from build123d import *

# Parameters (mm, degrees)
F1_DEPTH = 60


with BuildPart() as f1:
    # F0 (on Top) → F1 (new body)
    with BuildSketch(Plane.XY):
        with BuildLine():
            Line((-85, -85), (85, -85))
            Line((85, -85), (83.56066, -83.56066))
            ThreePointArc((83.56066, -83.56066), (81.43934, -83.56066), (81.43934, -81.43934))
            Line((81.43934, -81.43934), (80.000001, -80.000001))
            Line((80.000001, -80.000001), (-80.000001, -80.000001))
            Line((-80.000001, -80.000001), (-81.43934, -81.43934))
            ThreePointArc((-81.43934, -81.43934), (-81.114181, -81.925975), (-81, -82.5))
            ThreePointArc((-81, -82.5), (-81.925975, -83.88582), (-83.56066, -83.56066))
            Line((-83.56066, -83.56066), (-85, -85))
        make_face()
        with BuildLine():
            Line((-85, 85), (-85, -85))
            Line((-85, -85), (-83.56066, -83.56066))
            ThreePointArc((-83.56066, -83.56066), (-83.56066, -81.43934), (-81.43934, -81.43934))
            Line((-81.43934, -81.43934), (-80.000001, -80.000001))
            Line((-80.000001, -80.000001), (-80.000001, 80.000001))
            Line((-80.000001, 80.000001), (-81.43934, 81.43934))
            ThreePointArc((-81.43934, 81.43934), (-83.56066, 81.43934), (-83.56066, 83.56066))
            Line((-83.56066, 83.56066), (-85, 85))
        make_face()
        with BuildLine():
            Line((83.56066, -83.56066), (85, -85))
            Line((85, -85), (85, 85))
            Line((85, 85), (83.56066, 83.56066))
            ThreePointArc((83.56066, 83.56066), (83.88582, 83.074025), (84, 82.5))
            ThreePointArc((84, 82.5), (83.074025, 81.114181), (81.43934, 81.43934))
            Line((81.43934, 81.43934), (80.000001, 80.000001))
            Line((80.000001, 80.000001), (80.000001, -80.000001))
            Line((80.000001, -80.000001), (81.43934, -81.43934))
            ThreePointArc((81.43934, -81.43934), (83.074025, -81.114181), (84, -82.5))
            ThreePointArc((84, -82.5), (83.88582, -83.074025), (83.56066, -83.56066))
        make_face()
        with BuildLine():
            Line((83.56066, 83.56066), (85, 85))
            Line((85, 85), (-85, 85))
            Line((-85, 85), (-83.56066, 83.56066))
            ThreePointArc((-83.56066, 83.56066), (-81.925975, 83.88582), (-81, 82.5))
            ThreePointArc((-81, 82.5), (-81.114181, 81.925975), (-81.43934, 81.43934))
            Line((-81.43934, 81.43934), (-80.000001, 80.000001))
            Line((-80.000001, 80.000001), (80.000001, 80.000001))
            Line((80.000001, 80.000001), (81.43934, 81.43934))
            ThreePointArc((81.43934, 81.43934), (81.43934, 83.56066), (83.56066, 83.56066))
        make_face()
    extrude(amount=F1_DEPTH)


solid = f1.part
Verification items for the finished model (mm, model axes). A direction names the side the tool comes from. Give positions to 0.01 mm unless a question says otherwise; leave off trailing zeros. Loops run counter-clockwise (first coordinate to the right, second up) from the corner with the lowest first, then second, coordinate; pieces in that order, holes last.
1) Thickness scan on line 1 along X through (y, z) = (-67, 18.5). Record the ranges inside material, lowest first.
2) Sectioned sample at A-A, the plane x = -29.5. Enter the section's corners in (y, z).
3) Set-up check for faces 1 (the flat face through (0, 82, 60)), 2 (the flat face through (-1, 80, 30)): record each of +Z, -Z, +X, -X, +Y, -Y from which the full face is reachable in a straight line by a thin tool's end or side.
4) Sectioned sample at B-B, the plane z = 23. Enter the section's corners in (x, y).
5) Draft check along Y on faces 3 (the flat face through (-1, -85, 30)), 4 (the flat face through (1, -80, 30)), 5 (the flat face through (85, -1, 30)). Enter one of: pulls with the +Y half, pulls with the -Y half, needs draft (parallel to the pull), parting line crosses it, or undercut.
Answers:
1. line 1: x = -85 to -80, 80 to 85
2. outline: (-85, 0) - (-80, 0) - (-80, 60) - (-85, 60) - close; (80, 0) - (85, 0) - (85, 60) - (80, 60) - close
3. face 1: +Z, +X, -X, +Y, -Y
3. face 2: +Z, -Z
4. outline: (-85, -85) - (85, -85) - (85, 85) - (-85, 85) - close; hole (-83.56, -83.56) arc R1.5 ccw to (-81, -82.5) arc R1.5 ccw to (-81.44, -81.44) arc R1.5 ccw to start; hole (-83.56, 83.56) arc R1.5 ccw to (-81.44, 81.44) arc R1.5 ccw to (-81, 82.5) arc R1.5 ccw to start; hole (-80, -80) - (80, -80) - (80, 80) - (-80, 80) - close; hole (83.56, -83.56) arc R1.5 ccw to (84, -82.5) arc R1.5 ccw (long way) to start; hole (83.56, 83.56) arc R1.5 ccw (long way) to (84, 82.5) arc R1.5 ccw to start
5. face 3: pulls with the -Y half
5. face 4: undercut
5. face 5: needs draft
